Read the model definition and answer for the solid it produces. Units are mm, in the model's axes. A direction names the side the tool comes from. Coordinates: 2 decimals unless noted, no trailing zeros. Write each loop counter-clockwise with the first axis right and the second up, starting at its lowest first coordinate (ties: lowest second). Pieces come first, ordered by that corner, then holes. Notation, with made-up numbers: (-37, 62) -> (-33, 62) arc R14 ccw to (-33, 66) -> close; hole circle Ø9 at (-9, -35.5). An arc over 180 degrees is marked (long way). One line per item, written item: value. Start each with the question number.
1. Find section B-B, the plane x = 4.5. Write down the section's boundary in (y, z), and give its area (3 significant figures).
2. Find section C-C, the plane z = 19.5. Write down the section's boundary in (x, y), and give its area (3 significant figures).
3. Consider line 1 along X through (y, z) = (-1, 18); line 2 along Z through (x, y) = (0, -3.5); line 3 along Z through (x, y) = (-4.25, -13.5). Determine where each line is inside the solid, lowest interval first.
4. Find section D-D, the plane y = -3.5. Write down the section's boundary in (x, z), and give its area (3 significant figures).
5. For a pull along Z with two mould halves and no side action, classify faces 1 (the cylindrical face through (-2.48, -0.44, 29.97)), 2 (the flat face through (3.75, 0, 0)), 3 (the cylindrical face through (0.018, -5.878, 8.164)) as pulls with the +Z half, pulls with the -Z half, needs draft (parallel to the pull), parting line crosses it, or undercut.
6. Given P1, Ø3, axis at y = 0, z = 1, coming from the -X side; P2, Ø1, axis at x = -1, z = 16.5, coming from the -Y side; P3, Ø6, axis at x = 4.5, z = 12, coming from the -Y side; P4, Ø3, axis at y = -2.5, z = 22.5, coming from the +X side, each flat-ended and moving along its own axis, determine where each tip first touches the part or whether it passes through.
7. Find section A-A, the plane z = 10. Write down the section's boundary in (x, y).
8. For faces 4 (the cylindrical face through (-3.715, -14.285, 5.086)), 5 (the flat face through (-3.75, 0, 0)), 6 (the cylindrical face through (2.48, -0.44, 29.97)), determine the directions among +Z, -Z, +X, -X, +Y, -Y from which every point of the face is accessible in a straight line to the end or side of a thin tool.
```python
from build123d import *

# Parameters (mm, degrees)
EXTRUDE_1_DEPTH     = 1.25
SKETCH_1_3_R        = 2
CUT_EXTRUDE_1_DEPTH = 37.497164572
FILLET_1_R          = 3
EXTRUDE_START       = -1.25
SKETCH_2_R          = 2
EXTRUDE_2_DEPTH     = 1.25
SKETCH_2_5_R        = 1.8
EXTRUDE_5_DEPTH     = 2.5
SKETCH_2_7_R        = 1.8
EXTRUDE_7_DEPTH     = 5


with BuildPart() as part:
    # 草图1 → 凸台-拉伸1 (new body)
    with BuildSketch(Plane(origin=(0, 0, 0), x_dir=(0, 0, -1), z_dir=(1, 0, 0))):
        with BuildLine():
            Line((-28.172077255, -4.520836084), (-28.172077255, 1.479163916))
            Line((-28.172077255, 1.479163916), (-24.707975639, 1.479163916))
            ThreePointArc((-24.707975639, 1.479163916), (-31.63617887, 1.479163916), (-28.172077255, -4.520836084))
        make_face()
        with BuildLine():
            Line((-24.707975639, 1.479163916), (-28.172077255, 1.479163916))
            Line((-28.172077255, 1.479163916), (-28.172077255, -4.520836084))
            ThreePointArc((-28.172077255, -4.520836084), (-25.34365013, -3.349263209), (-24.172077255, -0.520836084))
            ThreePointArc((-24.172077255, -0.520836084), (-24.308373949, 0.514440097), (-24.707975639, 1.479163916))
        make_face()
        with BuildLine():
            Line((-3.172077255, 1.479163916), (-24.707975639, 1.479163916))
            ThreePointArc((-24.707975639, 1.479163916), (-24.308373949, 0.514440097), (-24.172077255, -0.520836084))
            ThreePointArc((-24.172077255, -0.520836084), (-25.34365013, -3.349263209), (-28.172077255, -4.520836084))
            Line((-28.172077255, -4.520836084), (-5.969923204, -4.520836084))
            Line((-5.969923204, -4.520836084), (-3.172077255, 1.479163916))
        make_face()
        with BuildLine():
            Line((3.172077255, -1.479163916), (-3.172077255, 1.479163916))
            Line((-3.172077255, 1.479163916), (-3.172077255, -1.479163916))
            ThreePointArc((-3.172077255, -1.479163916), (0, -3.5), (3.172077255, -1.479163916))
        make_face()
        with BuildLine():
            ThreePointArc((3.5, 0), (0.757538649, 3.417036025), (-3.172077255, 1.479163916))
            Line((-3.172077255, 1.479163916), (3.172077255, -1.479163916))
            ThreePointArc((3.172077255, -1.479163916), (3.417036025, -0.757538649), (3.5, 0))
        make_face()
        with BuildLine():
            ThreePointArc((-3.172077255, -1.479163916), (-3.5, 0), (-3.172077255, 1.479163916))
            Line((-3.172077255, 1.479163916), (-5.969923204, -4.520836084))
            Line((-5.969923204, -4.520836084), (-3.172077255, -4.520836084))
            Line((-3.172077255, -4.520836084), (-3.172077255, -1.479163916))
        make_face()
        with BuildLine():
            Line((-3.172077255, -1.479163916), (-3.172077255, 1.479163916))
            ThreePointArc((-3.172077255, 1.479163916), (-3.5, 0), (-3.172077255, -1.479163916))
        make_face()
        with BuildLine():
            Line((-3.172077255, -4.520836084), (-5.969923204, -4.520836084))
            Line((-5.969923204, -4.520836084), (-7.893387964, -8.645719574))
            ThreePointArc((-7.893387964, -8.645719574), (-4.014873487, -8.609923977), (-1.549233455, -11.604047406))
            Line((-1.549233455, -11.604047406), (3.172077255, -1.479163916))
            ThreePointArc((3.172077255, -1.479163916), (0, -3.5), (-3.172077255, -1.479163916))
            Line((-3.172077255, -1.479163916), (-3.172077255, -4.520836084))
        make_face()
        with BuildLine():
            ThreePointArc((-1.549233455, -11.604047406), (-4.014873487, -8.609923977), (-7.893387964, -8.645719574))
            Line((-7.893387964, -8.645719574), (-9.088732919, -11.209145102))
            Line((-9.088732919, -11.209145102), (-2.74457841, -14.167472935))
            Line((-2.74457841, -14.167472935), (-1.549233455, -11.604047406))
        make_face()
        with BuildLine():
            Line((-9.088732919, -11.209145102), (-7.893387964, -8.645719574))
            ThreePointArc((-7.893387964, -8.645719574), (-8.299375187, -16.50572276), (-1.416655664, -12.688309019))
            ThreePointArc((-1.416655664, -12.688309019), (-1.449923081, -12.14214052), (-1.549233455, -11.604047406))
            Line((-1.549233455, -11.604047406), (-2.74457841, -14.167472935))
            Line((-2.74457841, -14.167472935), (-9.088732919, -11.209145102))
        make_face()
    extrude(amount=EXTRUDE_1_DEPTH)

    # 草图1<3> → 切除-拉伸1 (cut, through all)
    with BuildSketch(Plane(origin=(0, 0, 0), x_dir=(0, 0, -1), z_dir=(1, 0, 0))):
        with Locations((-28.172077255, -0.520836084)):
            Circle(SKETCH_1_3_R)
        Circle(SKETCH_1_3_R)
        with Locations((-5.916655664, -12.688309019)):
            Circle(SKETCH_1_3_R)
    extrude(amount=CUT_EXTRUDE_1_DEPTH, mode=Mode.SUBTRACT)

    # 圆角1
    # the kernel refuses this fillet: 3 mm, written as the material it adds along each edge
    with BuildSketch(Plane(origin=(0, -11.604047406, 1.549233455), x_dir=(0, 0.9063077870366663, -0.4226182617406644), z_dir=(1, 0, 0))) as fillet_1_piece_1:
        with BuildLine():
            CenterArc((0.913230262, -3), FILLET_1_R, 90, 29.926434867)
            Line((-0.583432693, -0.4), (-0.613365952, -0.348))
            ThreePointArc((-0.613365952, -0.348), (-0.317772106, -0.161995545), (-0.037712362, 0.046666667))
            Line((-0.037712362, 0.046666667), (0, 0.06))
            Line((0, 0.06), (0.913230262, 0.06))
            Line((0.913230262, 0.06), (0.913230262, 0))
        make_face()
    extrude(amount=1.25)
    with BuildSketch(Plane(origin=(0, 1.479163916, 3.172077255), x_dir=(0, 0, 1), z_dir=(1, 0, 0))) as fillet_1_piece_2:
        with BuildLine():
            CenterArc((1.538240209, -3), FILLET_1_R, 90, 46.440922497)
            Line((-0.635752466, -0.932693577), (-0.67923232, -0.891347449))
            ThreePointArc((-0.67923232, -0.891347449), (-0.329607023, -0.458350724), (-0.054378467, 0.025357096))
            Line((-0.054378467, 0.025357096), (0, 0.06))
            Line((0, 0.06), (1.538240209, 0.06))
            Line((1.538240209, 0.06), (1.538240209, 0))
        make_face()
    extrude(amount=1.25)
    with BuildSketch(Plane(origin=(0, 1.479163916, 24.707975639), x_dir=(0, 0.7902368852402469, 0.6128014892326821), z_dir=(1, 0, 0))) as fillet_1_piece_3:
        with BuildLine():
            CenterArc((1.49141536, -2.972297887), FILLET_1_R, 97.792345701, 44.415308597)
            Line((-0.879295296, -1.133893419), (-0.926709509, -1.09712533))
            Line((-0.926709509, -1.09712533), (-0.047414213, 0.036768089))
            Line((-0.047414213, 0.036768089), (0.008134993, 0.059445958))
            ThreePointArc((0.008134993, 0.059445958), (0.542332858, 0.023063849), (1.076530723, 0.059445958))
            Line((1.076530723, 0.059445958), (1.084665716, 0))
        make_face()
    extrude(amount=1.25)
    with BuildSketch(Plane(origin=(0, -4.520836084, 5.969923204), x_dir=(0, 0, 1), z_dir=(1, 0, 0))) as fillet_1_piece_4:
        with BuildLine():
            CenterArc((4.704586321, 3), FILLET_1_R, 157.978087479, 112.021912521)
            Line((1.923464761, 4.12488349), (1.867842329, 4.14738116))
            ThreePointArc((1.867842329, 4.14738116), (0.907353913, 2.087798841), (-0.054378467, 0.025357096))
            Line((-0.054378467, 0.025357096), (0, -0.06))
            Line((0, -0.06), (4.704586321, -0.06))
            Line((4.704586321, -0.06), (4.704586321, 0))
        make_face()
    extrude(amount=1.25)

    # 草图2 → 凸台-拉伸2 (add)
    with BuildSketch(Plane(origin=(1.25, 0, 0), x_dir=(0, 0, -1), z_dir=(1, 0, 0)).offset(EXTRUDE_START)):
        Circle(SKETCH_2_R)
        with Locations((-5.916655664, -12.688309019)):
            Circle(SKETCH_2_R)
        with Locations((-28.172077255, -0.520836084)):
            Circle(SKETCH_2_R)
    extrude(amount=EXTRUDE_2_DEPTH)

    # 草图2<5> → 凸台-拉伸5 (add)
    with BuildSketch(Plane(origin=(1.25, 0, 0), x_dir=(0, 0, -1), z_dir=(1, 0, 0))):
        with Locations((-28.172077255, -0.520836084)):
            Circle(SKETCH_2_5_R)
        Circle(SKETCH_2_5_R)
    extrude(amount=EXTRUDE_5_DEPTH)

    # 草图2<7> → 凸台-拉伸7 (add)
    with BuildSketch(Plane(origin=(1.25, 0, 0), x_dir=(0, 0, -1), z_dir=(1, 0, 0))):
        with Locations((-5.916655664, -12.688309019)):
            Circle(SKETCH_2_7_R)
    extrude(amount=EXTRUDE_7_DEPTH)

    # 镜向1: part across plane


with BuildPart() as part_1:
    add(part.part)
    add(part.part.mirror(Plane.ZY))


solid = part_1.part
```
Answer block:
1. outline: circle Ø3.6 at (-12.69, 5.92)
1. area: 10.2 mm2
2. outline: (-1.25, -4.52) -> (1.25, -4.52) -> (1.25, 1.48) -> (-1.25, 1.48) -> close
2. area: 15.0 mm2
3. line 1: x = -1.25 to 1.25
3. line 2: z = -2.23 to 30.84
3. line 3: z = 4.31 to 7.52
4. outline: (-1.25, -2.23) -> (1.25, -2.23) -> (1.25, 30.84) -> (-1.25, 30.84) -> close
4. area: 82.7 mm2
5. face 1: undercut
5. face 2: needs draft
5. face 3: pulls with the +Z half
6. P1: stops at x = -3.75
6. P2: stops at y = -4.52
6. P3: passes through
6. P4: stops at x = 1.25
7. outline: (-1.25, -14.58) -> (1.25, -14.58) -> (1.25, -10.8) -> (-1.25, -10.8) -> close; (-1.25, -4.6) -> (1.25, -4.6) -> (1.25, 1.48) -> (-1.25, 1.48) -> close
8. face 4: -X
8. face 5: +Z, -Z, -X, +Y, -Y
8. face 6: +X
